from build123d import *

# Parameters (mm, degrees)
SKETCH_1_W          = 25
SKETCH_1_H          = 50
EXTRUDE_1_DEPTH     = 2214.15898255
CUT_EXTRUDE_2_DEPTH = 50
CUT_EXTRUDE_3_DEPTH = 50


with BuildPart() as part:
    # Эскиз1 → Бобышка-Вытянуть1 (new body)
    with BuildSketch(Plane(origin=(0, 0, 0), x_dir=(1, 0, 0), z_dir=(0, 1, 0))):
        Rectangle(SKETCH_1_W, SKETCH_1_H)
    extrude(amount=EXTRUDE_1_DEPTH)

    # Эскиз3 → Вырез-Вытянуть2 (cut)
    with BuildSketch(Plane.ZY.offset(12.5)):
        Polygon((25, 0), (-25, 105.257973095), (-25, 0), align=None)
    extrude(amount=-CUT_EXTRUDE_2_DEPTH, mode=Mode.SUBTRACT)

    # Эскиз4 → Вырез-Вытянуть3 (cut)
    with BuildSketch(Plane.ZY.offset(12.5)):
        Polygon((25, 2214.15898255), (-25, 2190.418247515), (-25, 2214.15898255), align=None)
    extrude(amount=-CUT_EXTRUDE_3_DEPTH, mode=Mode.SUBTRACT)


solid = part.part
Verification items for the finished model (mm, model axes). Round coordinates to 2 decimals unless told otherwise and drop trailing zeros. Write each loop counter-clockwise with the first axis right and the second up, starting at its lowest first coordinate (ties: lowest second). Pieces come first, ordered by that corner, then holes.
(1) Section check A-A (x = -7.5). Enter the section's corners in (y, z), plus the area to 3 significant figures.
Returned:
outline: (0, 25) - (105.26, -25) - (2190.42, -25) - (2214.16, 25) - close
area: 107,000 mm2
(2) Section check B-B (z = -8). Enter the section's corners in (x, y).
Returned:
outline: (-12.5, 69.47) - (12.5, 69.47) - (12.5, 2198.49) - (-12.5, 2198.49) - close
(3) Depth check by flat-ended pin: pin 1 Ø10 at (x, z) = (-4.5, 19.5) entering from -Y; pin 2 Ø12 at (x, z) = (-9, 8) entering from -Y; pin 3 Ø12 at (x, z) = (8.5, -1.5) entering from -Y. Enter the tip coordinate at first touch or a pass-through.
Returned:
pin 1: stops at y = 1.05
pin 2: stops at y = 23.16
pin 3: stops at y = 43.16
(4) Material ranges on line 1 (Y direction, x = 11, z = 13); line 2 (Y direction, x = 10, z = 16), recorded low to high.
Returned:
line 1: y = 25.26 to 2208.46
line 2: y = 18.95 to 2209.89
